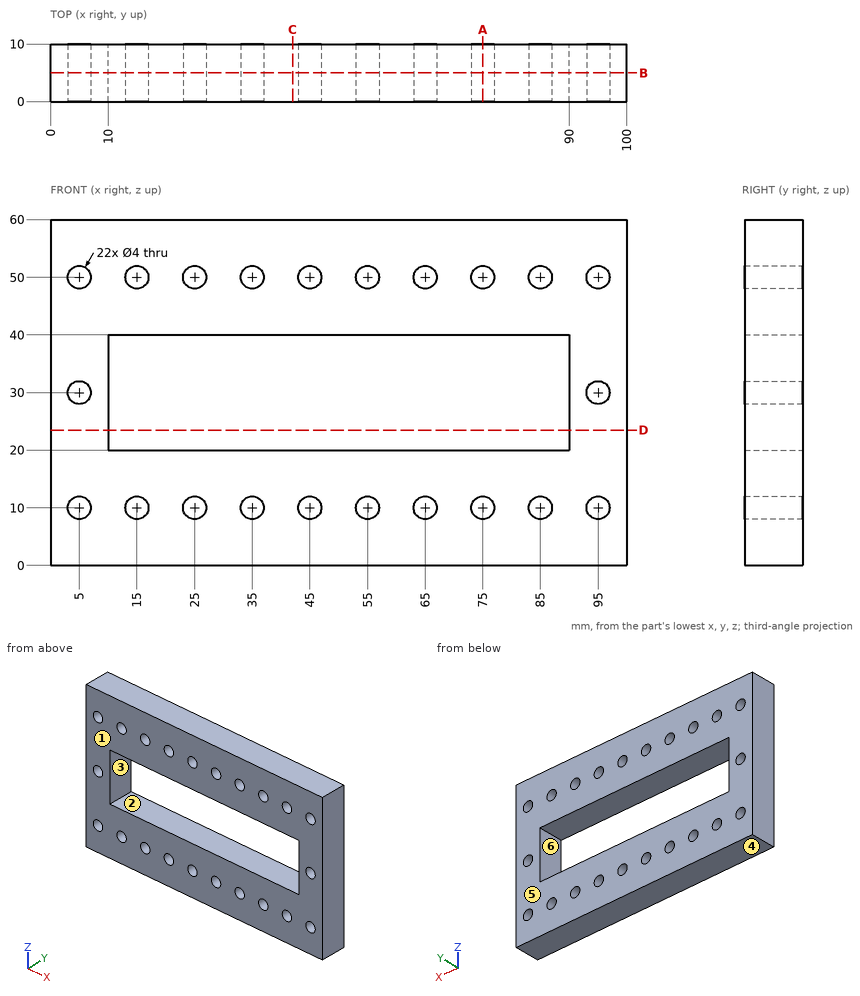
Verification items for this drawing (mm, ordinates from the low corner). A direction names the side the tool comes from. Give positions to 0.01 mm unless a question says otherwise; leave off trailing zeros. Write each loop counter-clockwise with the first axis right and the second up, starting at its lowest first coordinate (ties: lowest second). Pieces come first, ordered by that corner, then holes. Notation, with made-up numbers: (61.25, 33) - (101.25, 33) arc R23 ccw to (101.25, 42) - close; hole circle Ø8 at (-19, 86). An arc over 180 degrees is marked (long way). Answer as a JSON object with one key per item and string values. Group by question number.
1) Sectioned sample at B-B (y = 5). Give the number of separate pieces and of enclosed holes in the cut face, then the cut area to 3 significant figures.
2) Sectioned sample at D-D (z = 23.5). Record the cut outline in (x, y).
3) Thickness scan on probe 1 along Z at (x, y) = (68.5, 1.75); probe 2 along Z at (x, y) = (74.5, 3). Record the ranges inside material, lowest first. Write a range as from..to.
4) Sectioned sample at A-A (x = 75). Record the cut outline in (y, z), then the cut area to 3 significant figures.
5) Sectioned sample at C-C (x = 42). Record the cut outline in (y, z).
6) Access from +Z, -Z, +X, -X, +Y, -Y to the whole of each face (thin tool, end or side, straight path). Record for the marked faces 5 and 6.
7) Release check for a two-part mould opening along Z. For the marked faces 1, 2, 3 and 4 record: pulls with the +Z half, pulls with the -Z half, needs draft (parallel to the pull), parting line crosses it, or undercut.
8) Depth check by flat-ended pin: P1, Ø1, axis at x = 34.5, z = 49.5, coming from the +Y side; P2, Ø3, axis at x = 34, y = 4.5, coming from the -Z side. Enter the tip coordinate at first touch or a pass-through.
Geometry results:
{
 "1": {"separate pieces": "1", "enclosed holes": "23", "area": "4,120 mm^2"},
 "2": {"outline": "(0, 0) - (10, 0) - (10, 10) - (0, 10) - close; (90, 0) - (100, 0) - (100, 10) - (90, 10) - close"},
 "3": {"probe 1": "z = 0..20, 40..60", "probe 2": "z = 0..8.06, 11.94..20, 40..48.06, 51.94..60"},
 "4": {"outline": "(0, 0) - (10, 0) - (10, 8) - (0, 8) - close; (0, 12) - (10, 12) - (10, 20) - (0, 20) - close; (0, 40) - (10, 40) - (10, 48) - (0, 48) - close; (0, 52) - (10, 52) - (10, 60) - (0, 60) - close", "area": "320 mm^2"},
 "5": {"outline": "(0, 0) - (10, 0) - (10, 20) - (0, 20) - close; (0, 40) - (10, 40) - (10, 60) - (0, 60) - close"},
 "6": {"face 5": "+Z, -Z, +X, -X, +Y", "face 6": "+Y, -Y"},
 "7": {"face 1": "needs draft", "face 2": "undercut", "face 3": "undercut", "face 4": "pulls with the -Z half"},
 "8": {"P1": "passes through", "P2": "stops at z = 0"}
}
